from build123d import *

# Parameters (mm, degrees)
P_IDAT_VYSUNUT_M1_DEPTH  = 5
SKICA2_R                 = 2.5
ODEBRAT_VYSUNUT_M1_DEPTH = 5
ODEBRAT_VYSUNUT_M2_DEPTH = 5
P_IDAT_VYSUNUT_M2_DEPTH  = 5


with BuildPart() as part:
    # Skica1 → Přidat vysunutím1 (new body)
    with BuildSketch(Plane.XY):
        Polygon((-91.646058289, -95), (91.646058289, -95), (91.646058289, -30), (0, 15), (-91.646058289, -30), align=None)
    extrude(amount=P_IDAT_VYSUNUT_M1_DEPTH)

    # Skica2 → Odebrat vysunutím1 (cut)
    with BuildSketch(Plane.XY.offset(5)):
        Circle(SKICA2_R)
    extrude(amount=-ODEBRAT_VYSUNUT_M1_DEPTH, mode=Mode.SUBTRACT)

    # Skica3 → Odebrat vysunutím2 (cut)
    with BuildSketch(Plane.XY.offset(5)):
        Polygon((91.646058289, -30), (15, -30), (15, 7.634707781), align=None)
        Polygon((-15, 7.634707781), (-91.646058289, -30), (-15, -30), align=None)
    extrude(amount=-ODEBRAT_VYSUNUT_M2_DEPTH, mode=Mode.SUBTRACT)

    # Skica4 → Přidat vysunutím2 (add)
    with BuildSketch(Plane.XY.offset(5)):
        with BuildLine():
            Line((-91.646058289, -95), (91.646058289, -95))
            ThreePointArc((91.646058289, -95), (0, -118.848037221), (-91.646058289, -95))
        make_face()
    extrude(amount=-P_IDAT_VYSUNUT_M2_DEPTH)


solid = part.part
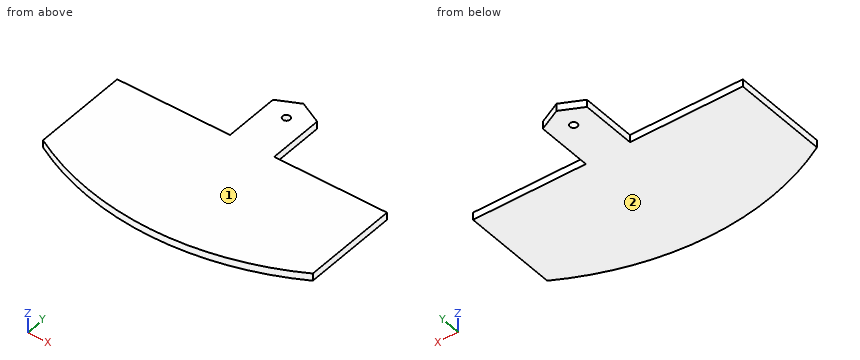
Read the model definition and answer for the solid it produces. Units are mm, in the model's axes. Face numbers are marked on the shaded views. Give positions to 0.01 mm unless a question says otherwise; leave off trailing zeros. Loops run counter-clockwise (first coordinate to the right, second up) from the corner with the lowest first, then second, coordinate; pieces in that order, holes last. Notation, with made-up numbers: (27.5, -13) -> (41.5, -13) arc R34 cw to (41.5, 17) -> close; hole circle Ø6 at (2.5, -35.5). An arc over 180 degrees is marked (long way). Use a Markdown table: item, result.
Q1. Section C-C, the plane x = -57 is taken. Determine the outline of the cut face in (y, z).
Solved:
| item | result |
|---|---|
| outline | (-110, 0) -> (-30, 0) -> (-30, 5) -> (-110, 5) -> close |
Q2. Find the intervals of material crossed by line 1 along Y through (x, z) = (0, 1.7); line 2 along X through (y, z) = (-12.5, 0.3); line 3 along Y through (x, z) = (34.5, 4.55), in increasing order.
Solved:
| item | result |
|---|---|
| line 1 | y = -118.85 to -2.5, 2.5 to 15 |
| line 2 | x = -15 to 15 |
| line 3 | y = -115.66 to -30 |
Q3. Section D-D, the plane x = -38 is taken. Determine the outline of the cut face in (y, z), then the cut area to 3 significant figures.
Solved:
| item | result |
|---|---|
| outline | (-114.97, 0) -> (-30, 0) -> (-30, 5) -> (-114.97, 5) -> close |
| area | 425 mm^2 |
Q4. Each of these flat-tipped pins is pushed along its axis until it touches: pin 1 (2 mm diameter, centred on y = -27, z = 0.5, fed in from -X); pin 2 (1.5 mm diameter, centred on x = -51, z = 1.5, fed in from -Y). Where does it stop, or does it pass through?
Solved:
| item | result |
|---|---|
| pin 1 | stops at x = -15 |
| pin 2 | stops at y = -112.01 |
Q5. Section B-B, the plane z = 1.65 is taken. Determine the outline of the cut face in (x, y), then the cut area to 3 significant figures.
Solved:
| item | result |
|---|---|
| outline | (-91.65, -95) arc R188.02 ccw to (91.65, -95) -> (91.65, -30) -> (15, -30) -> (15, 7.63) -> (0, 15) -> (-15, 7.63) -> (-15, -30) -> (-91.65, -30) -> close; hole circle Ø5 at (0, 0) |
| area | 16,100 mm^2 |
Q6. Determine the mould class of the marked faces 1 and 2 for opening direction Z: pulls with the +Z half, pulls with the -Z half, needs draft (parallel to the pull), parting line crosses it, or undercut.
Solved:
| item | result |
|---|---|
| face 1 | pulls with the +Z half |
| face 2 | pulls with the -Z half |
Q7. Section A-A, the plane y = 0 is taken. Determine the outline of the cut face in (x, z), then the cut area to 3 significant figures.
Solved:
| item | result |
|---|---|
| outline | (-15, 0) -> (-2.5, 0) -> (-2.5, 5) -> (-15, 5) -> close; (2.5, 0) -> (15, 0) -> (15, 5) -> (2.5, 5) -> close |
| area | 125 mm^2 |
